Here's how the part is built. I have some questions about the finished solid (model axes, mm). A direction names the side the tool comes from. Give positions to 0.01 mm unless a question says otherwise; leave off trailing zeros. Loops run counter-clockwise (first coordinate to the right, second up) from the corner with the lowest first, then second, coordinate; pieces in that order, holes last. Notation, with made-up numbers: (42.25, 53) - (48.25, 53) arc R22 ccw to (48.25, 63) - close; hole circle Ø2 at (-17, 17.5). An arc over 180 degrees is marked (long way). Put each result on its own line as item: value. Start each with the question number.
from build123d import *

# Parameters (mm, degrees)
SKETCH1_R                = 12.15
SKETCH1_R_2              = 9.15
BOSS_EXTRUDE1_DEPTH      = 10
BOSS_EXTRUDE2_DEPTH      = 2.1
BOSS_EXTRUDE2_DEPTH_BACK = 2.1
SKETCH4_W                = 4.2
SKETCH4_H                = 10
BOSS_EXTRUDE3_DEPTH      = 53
FILLET1_R                = 12
SKETCH5_R                = 14.2
SKETCH5_R_2              = 11.2
BOSS_EXTRUDE4_DEPTH      = 50.547009
BOSS_EXTRUDE11_DEPTH     = 4.2
BOSS_EXTRUDE12_DEPTH     = 4.2
FILLET2_R                = 6
FILLET3_R                = 2
SKETCH10_R               = 11.2
CUT_EXTRUDE2_DEPTH       = 51.547008827
SKETCH15_R               = 1.7
CUT_EXTRUDE5_DEPTH       = 1
CUT_EXTRUDE5_DEPTH_BACK  = 29.4
SKETCH17_R               = 2.9
CUT_EXTRUDE6_DEPTH       = 1.5
CUT_EXTRUDE7_DEPTH       = 1.5
SKETCH19_W               = 28
SKETCH19_H               = 17
CUT_EXTRUDE8_DEPTH       = 26.4000001
CUT_EXTRUDE8_DEPTH_BACK  = 4


with BuildPart() as part:
    # Sketch1 → Boss-Extrude1 (new body)
    with BuildSketch(Plane.XY):
        Circle(SKETCH1_R)
        Circle(SKETCH1_R_2, mode=Mode.SUBTRACT)
    extrude(amount=BOSS_EXTRUDE1_DEPTH)

    # Sketch2 → Boss-Extrude2 (add, two sides)
    with BuildSketch(Plane.XY.offset(5)) as boss_extrude2_sk:
        with BuildLine():
            Line((11.073504414, 5), (21.073504414, 5))
            Line((21.073504414, 5), (21.073504414, -5))
            Line((21.073504414, -5), (11.073504414, -5))
            ThreePointArc((11.073504414, -5), (12.15, 0), (11.073504414, 5))
        make_face()
        with BuildLine():
            ThreePointArc((-11.073504414, 5), (-12.15, 0), (-11.073504414, -5))
            Line((-11.073504414, -5), (-21.073504414, -5))
            Line((-21.073504414, -5), (-21.073504414, 5))
            Line((-21.073504414, 5), (-11.073504414, 5))
        make_face()
    extrude(amount=BOSS_EXTRUDE2_DEPTH)
    extrude(boss_extrude2_sk.sketch, amount=-BOSS_EXTRUDE2_DEPTH_BACK)

    # Sketch4 → Boss-Extrude3 (add)
    with BuildSketch(Plane(origin=(0, 0, 2.9), x_dir=(-1, 0, 0), z_dir=(0, 0, -1))):
        with Locations((23.173504414, 0)):
            Rectangle(SKETCH4_W, SKETCH4_H)
        with Locations((-23.173504414, 0)):
            Rectangle(SKETCH4_W, SKETCH4_H)
    extrude(amount=-BOSS_EXTRUDE3_DEPTH)

    # Fillet1
    fillet1_edges = [part.edges().sort_by_distance(p)[0] for p in [
        (11.073504414, 5, 5),
        (11.073504414, -5, 5),
        (-11.073504414, 5, 5),
        (-11.073504414, -5, 5),
    ]]
    fillet(fillet1_edges, radius=FILLET1_R)



with BuildPart() as body_2:
    # Sketch5 → Boss-Extrude4 (new body)
    with BuildSketch(Plane.ZY.offset(25.273504414)):
        with Locations((67.1, 0)):
            Circle(SKETCH5_R)
        with Locations((67.1, 0)):
            Circle(SKETCH5_R_2, mode=Mode.SUBTRACT)
    extrude(amount=-BOSS_EXTRUDE4_DEPTH)


with BuildPart() as part_1:
    add(part.part)

    add(body_2.part)  # Boss-Extrude11 merges body 2
    # Sketch7 → Boss-Extrude11 (add)
    with BuildSketch(Plane.ZY.offset(25.273504414)):
        with BuildLine():
            Line((56.60689185, -9.567375887), (56.60689185, 9.567375887))
            ThreePointArc((56.60689185, 9.567375887), (51.915920178, 6.192643958), (46.261573956, 5))
            Line((46.261573956, 5), (46.261573956, -5))
            ThreePointArc((46.261573956, -5), (51.915920178, -6.192643958), (56.60689185, -9.567375887))
        make_face()
    extrude(amount=-BOSS_EXTRUDE11_DEPTH)

    # Sketch9 → Boss-Extrude12 (add)
    with BuildSketch(Plane(origin=(25.273504414, 0, 0), x_dir=(0, 0, -1), z_dir=(1, 0, 0))):
        with BuildLine():
            Line((-56.60689185, 9.567375887), (-56.60689185, -9.567375887))
            ThreePointArc((-56.60689185, -9.567375887), (-51.915920178, -6.192643958), (-46.261573956, -5))
            Line((-46.261573956, -5), (-46.261573956, 5))
            ThreePointArc((-46.261573956, 5), (-51.915920178, 6.192643958), (-56.60689185, 9.567375887))
        make_face()
    extrude(amount=-BOSS_EXTRUDE12_DEPTH)

    # Fillet2
    fillet2_edges = [part_1.edges().sort_by_distance(p)[0] for p in [
        (-25.273504414, 0, 2.9),
        (25.273504414, 0, 2.9),
    ]]
    fillet(fillet2_edges, radius=FILLET2_R)

    # Fillet3
    fillet3_edges = [part_1.edges().sort_by_distance(p)[0] for p in [
        (21.073504414, 0, 7.1),
        (-21.073504414, 0, 7.1),
    ]]
    fillet(fillet3_edges, radius=FILLET3_R)

    # Sketch10 → Cut-Extrude2 (cut, through all)
    with BuildSketch(Plane(origin=(25.273504414, 0, 0), x_dir=(0, 0, -1), z_dir=(1, 0, 0))):
        with Locations((-67.1, 0)):
            Circle(SKETCH10_R)
    extrude(amount=-CUT_EXTRUDE2_DEPTH, mode=Mode.SUBTRACT)

    # Sketch15 → Cut-Extrude5 (cut, two sides)
    with BuildSketch(Plane(origin=(0, -14.2, 0), x_dir=(-1, 0, 0), z_dir=(0, -1, 0))) as cut_extrude5_sk:
        with Locations((-18.873504414, -67.1)):
            Circle(SKETCH15_R)
        with Locations((18.873504414, -67.1)):
            Circle(SKETCH15_R)
    extrude(amount=CUT_EXTRUDE5_DEPTH, mode=Mode.SUBTRACT)
    extrude(cut_extrude5_sk.sketch, amount=-CUT_EXTRUDE5_DEPTH_BACK, mode=Mode.SUBTRACT)

    # Sketch17 → Cut-Extrude6 (cut)
    with BuildSketch(Plane(origin=(0, -14.2, 0), x_dir=(-1, 0, 0), z_dir=(0, -1, 0))):
        with Locations((-18.873504414, -67.1)):
            Circle(SKETCH17_R)
        with Locations((18.873504414, -67.1)):
            Circle(SKETCH17_R)
    extrude(amount=-CUT_EXTRUDE6_DEPTH, mode=Mode.SUBTRACT)

    # Sketch18 → Cut-Extrude7 (cut)
    with BuildSketch(Plane(origin=(0, 14.2, 0), x_dir=(1, 0, 0), z_dir=(0, 1, 0))):
        Polygon((-15.873504414, -68.832050808), (-15.873504414, -65.367949192), (-18.873504414, -63.635898385), (-21.873504414, -65.367949192), (-21.873504414, -68.832050808), (-18.873504414, -70.564101615), align=None)
        Polygon((21.873504414, -68.832050808), (21.873504414, -65.367949192), (18.873504414, -63.635898385), (15.873504414, -65.367949192), (15.873504414, -68.832050808), (18.873504414, -70.564101615), align=None)
    extrude(amount=-CUT_EXTRUDE7_DEPTH, mode=Mode.SUBTRACT)

    # Sketch19 → Cut-Extrude8 (cut, two sides)
    with BuildSketch(Plane.XY.offset(55.9)) as cut_extrude8_sk:
        Rectangle(SKETCH19_W, SKETCH19_H)
    extrude(amount=CUT_EXTRUDE8_DEPTH, mode=Mode.SUBTRACT)
    extrude(cut_extrude8_sk.sketch, amount=-CUT_EXTRUDE8_DEPTH_BACK, mode=Mode.SUBTRACT)


solid = part_1.part
1) Thinking about a two-plate mould opening in Z: for faces 1 (the cylindrical face through (19.095, 11.874, 65.414)), 2 (the cylindrical face through (23.47, 0.07, 4.61)), 3 (the flat face through (14, 0, 79)), which applies, pulls with the +Z half, pulls with the -Z half, needs draft (parallel to the pull), parting line crosses it, or undercut?
2) I'm going to push flat-ended pins straight in: P1, Ø9, axis at x = -23, z = 20.5, coming from the -Y side; P2, Ø1, axis at x = -8, y = 11, coming from the -Z side; P3, Ø2, axis at x = 19, z = 8.5, coming from the +Y side; P4, Ø4, axis at x = -18.87, z = 67.1, coming from the +Y side. Where does each tip first touch, or does it pass through?
3) Which directions (+Z, -Z, +X, -X, +Y, -Y) give clear straight access to the entire face, cutting with the end or side of a thin tool? Please do faces 4 (the flat face through (23, 5, 25)), 5 (the cylindrical face through (-20.5, 0.1, 7.7)), 6 (the flat face through (-21.874, 13, 67)), 7 (the cylindrical face through (-12.47, 5.95, 5.03)).
4) Suppose I cut it at C-C on x = -10. Please give me the cut outline in (y, z), plus the area to 3 significant figures.
5) Suppose I cut it at A-A on x = 0. Please give me the cut outline in (y, z), plus the area to 3 significant figures.
6) Suppose I cut it at D-D on z = 67.1. Give the number of separate pieces and of enclosed holes in the cut face, plus the area to 3 significant figures.
7) Suppose I cut it at B-B on z = 18.5. Please give me the cut outline in (x, y), plus the area to 3 significant figures.
8) I need wall thicknesses on line 1 (X direction, y = -13, z = 67.1); line 2 (Z direction, x = -17, y = -0.25); line 3 (X direction, y = -11.65, z = 67.1). Which ranges of each line are inside material? Lowest first, please.
Ans:
1. face 1: undercut
1. face 2: pulls with the -Z half
1. face 3: needs draft
2. P1: stops at y = -5
2. P2: stops at z = 57.54
2. P3: passes through
2. P4: stops at y = 12.7
3. face 4: -Z, +X, +Y
3. face 5: +Y, -Y
3. face 6: +Y
3. face 7: -Z, -X, +Y
4. outline: (-8.5, 55.73) - (-8.5, 59.81) arc R11.2 cw to (-8.5, 74.39) - (-8.5, 78.47) arc R14.2 ccw to start; (-7.36, 2.9) - (-6.9, 2.9) - (-6.9, 0) - (6.9, 0) - (6.9, 2.9) - (7.36, 2.9) - (7.36, 7.1) - (6.9, 7.1) - (6.9, 10) - (-6.9, 10) - (-6.9, 7.1) - (-7.36, 7.1) - close; (8.5, 55.73) arc R14.2 ccw to (8.5, 78.47) - (8.5, 74.39) arc R11.2 cw to (8.5, 59.81) - close
4. area: 269 mm²
5. outline: (-12.15, 0) - (-9.15, 0) - (-9.15, 10) - (-12.15, 10) - close; (-8.5, 55.73) - (-8.5, 59.81) arc R11.2 cw to (-8.5, 74.39) - (-8.5, 78.47) arc R14.2 ccw to start; (8.5, 55.73) arc R14.2 ccw to (8.5, 78.47) - (8.5, 74.39) arc R11.2 cw to (8.5, 59.81) - close; (9.15, 0) - (12.15, 0) - (12.15, 10) - (9.15, 10) - close
5. area: 187 mm²
6. separate pieces: 6
6. enclosed holes: 0
6. area: 247 mm²
7. outline: (-25.27, -5) - (-21.07, -5) - (-21.07, 5) - (-25.27, 5) - close; (21.07, -5) - (25.27, -5) - (25.27, 5) - (21.07, 5) - close
7. area: 84.0 mm²
8. line 1: x = -25.27 to -21.77, -15.97 to 15.97, 21.77 to 25.27
8. line 2: z = 2.9 to 7.1, 52.9 to 55.9, 78.3 to 81.3
8. line 3: x = -25.27 to -20.57, -17.17 to 17.17, 20.57 to 25.27
